Here's how the part is built. I have some questions about the finished solid (model axes, mm). Face numbers are marked on the shaded views. A direction names the side the tool comes from. Coordinates: 2 decimals unless noted, no trailing zeros. Write each loop counter-clockwise with the first axis right and the second up, starting at its lowest first coordinate (ties: lowest second). Pieces come first, ordered by that corner, then holes. Notation, with made-up numbers: (28, 52) -> (60, 52) arc R26 cw to (60, 68) -> close; hole circle Ø6 at (-25, -1.75). An arc over 180 degrees is marked (long way). Use a Markdown table: item, result. Add a question column.
Item 1: Imagine slicing it at C-C, the plane z = 17. Write out the boundary of the cut face in (x, y), and give its area (3 significant figures).
Item 2: If I drill on line 1 along Y through (x, z) = (13.5, 2.05); line 2 along Z through (x, y) = (-10.5, 32); line 3 along X through (y, z) = (31.5, 4), over which ranges is the centre line in solid material (lowest first)? Write a range as from..to.
Item 3: Imagine slicing it at B-B, the plane x = 10. Write out the boundary of the cut face in (y, z), and give its area (3 significant figures).
Item 4: On a 3-axis mill with a long thin cutter (end or side, diameter ignored), from which of +Z, -Z, +X, -X, +Y, -Y can I reach the whole of each face in a straight line? I mean the marked faces 1 and 2. Say none if no direction works.
Item 5: Imagine slicing it at D-D, the plane z = 5. Write out the boundary of the cut face in (x, y).
Item 6: Imagine slicing it at A-A, the plane y = 42. Write out the boundary of the cut face in (x, z), and give its area (3 significant figures).
Item 7: Will these pins go through, and if not, where does the flat tip stop? pin 1 Ø1.4 at (x, y) = (7.5, 17) entering from -Z; pin 2 Ø4.5 at (x, y) = (-13.5, 0) entering from +Z; pin 3 Ø0.6 at (x, z) = (18.5, 11.5) entering from -Y; pin 4 Ø5 at (x, z) = (5, 8) entering from -Y.
```python
from build123d import *

# Parameters (mm, degrees)
SKETCH1_R           = 1.65
BOSS_EXTRUDE1_DEPTH = 3
BOSS_EXTRUDE2_DEPTH = 40
CHAMFER1_SIZE       = 3
CUT_EXTRUDE3_START  = -29
SKETCH4_W           = 14.985281374
SKETCH4_H           = 16.743157806
SKETCH4_W_2         = 6.029437252
CUT_EXTRUDE3_DEPTH  = 29
CUT_EXTRUDE4_DEPTH  = 86
CUT_EXTRUDE5_DEPTH  = 6


with BuildPart() as part:
    # Sketch1 → Boss-Extrude1 (new body)
    with BuildSketch(Plane.XY):
        Polygon((-20, 104), (-20, -4), (-9.014718626, -4), (-5.014718626, 0), (5.014718626, 0), (9.014718626, -4), (20, -4), (20, 104), (9.014718626, 104), (5.014718626, 100), (-5.014718626, 100), (-9.014718626, 104), align=None)
        with Locations((-13.5, 100)):
            Circle(SKETCH1_R, mode=Mode.SUBTRACT)
        with Locations((-13.5, 0)):
            Circle(SKETCH1_R, mode=Mode.SUBTRACT)
        with Locations(Location((13.5, 0, 0), (0, 0, 180))):
            Circle(SKETCH1_R, mode=Mode.SUBTRACT)
        with Locations(Location((13.5, 100, 0), (0, 0, 180))):
            Circle(SKETCH1_R, mode=Mode.SUBTRACT)
    extrude(amount=BOSS_EXTRUDE1_DEPTH)

    # Sketch2 → Boss-Extrude2 (add, through all)
    with BuildSketch(Plane.ZY.offset(20)):
        Polygon((3, 0), (32, 16.743157806), (32, 49.770526581), (3, 100), align=None)
    extrude(amount=-BOSS_EXTRUDE2_DEPTH)

    # Chamfer1
    chamfer1_edges = [part.edges().sort_by_distance(p)[0] for p in [
        (20, 33.256842194, 32),
        (-20, 33.256842194, 32),
    ]]
    chamfer(chamfer1_edges, length=CHAMFER1_SIZE)

    # Sketch4 → Cut-Extrude3 (cut)
    with BuildSketch(Plane.XY.offset(32).offset(CUT_EXTRUDE3_START)):
        with Locations((-12.507359313, 8.371578903)):
            Rectangle(SKETCH4_W, SKETCH4_H)
        with Locations((12.507359313, 8.371578903)):
            Rectangle(SKETCH4_W, SKETCH4_H)
        with Locations((0, 8.371578903)):
            Rectangle(SKETCH4_W_2, SKETCH4_H)
    extrude(amount=CUT_EXTRUDE3_DEPTH, mode=Mode.SUBTRACT)

    # Sketch5 → Cut-Extrude4 (cut)
    with BuildSketch(Plane(origin=(0, 104, 0), x_dir=(1, 0, 0), z_dir=(0, 1, 0))):
        Polygon((18, -3), (18, -28.171572875), (16.171572875, -30), (-16.171572875, -30), (-18, -28.171572875), (-18, -3), align=None)
    extrude(amount=-CUT_EXTRUDE4_DEPTH, mode=Mode.SUBTRACT)

    # Sketch6 → Cut-Extrude5 (cut)
    with BuildSketch(Plane(origin=(0, 16.743157806, 0), x_dir=(-1, 0, 0), z_dir=(0, -1, 0))):
        Polygon((5.014718626, -29), (15.757359313, -29), (18.757359313, -26), (20.757359313, -26), (20.757359313, -3), (5.014718626, -3), align=None)
        Polygon((-5.014718626, -3), (-5.014718626, -29), (-15.757359313, -29), (-18.757359313, -26), (-20.757359313, -26), (-20.757359313, -3), align=None)
    extrude(amount=-CUT_EXTRUDE5_DEPTH, mode=Mode.SUBTRACT)


solid = part.part
```
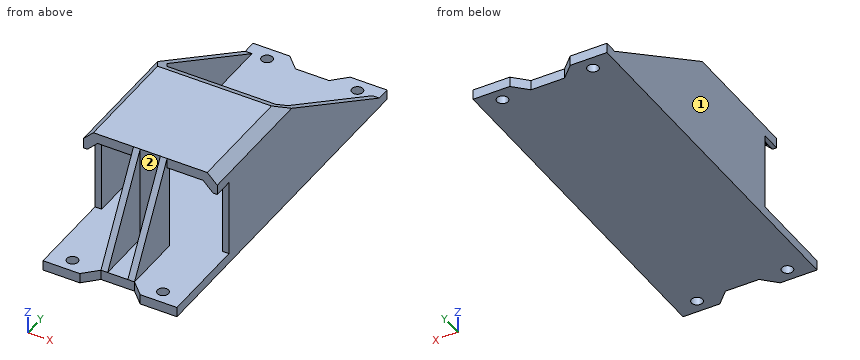
Ans:
| question | item | result |
|---|---|---|
| 1 | outline | (-20, 22.74) -> (-18, 22.74) -> (-18, 75.75) -> (-20, 75.75) -> close; (-5.01, 8.08) -> (-3.01, 8.08) -> (-3.01, 16.74) -> (3.01, 16.74) -> (3.01, 8.08) -> (5.01, 8.08) -> (5.01, 18) -> (-5.01, 18) -> close; (18, 22.74) -> (20, 22.74) -> (20, 75.75) -> (18, 75.75) -> close |
| 1 | area | 259 mm^2 |
| 2 | line 1 | y = -4..-1.65, 1.65..98.35, 101.65..104 |
| 2 | line 2 | z = 0..3, 30..32 |
| 2 | line 3 | x = -20..-18, 18..20 |
| 3 | outline | (-4, 0) -> (104, 0) -> (104, 3) -> (-4, 3) -> close; (16.74, 29) -> (18, 29) -> (18, 30) -> (53.23, 30) -> (49.77, 32) -> (16.74, 32) -> close |
| 3 | area | 395 mm^2 |
| 4 | face 1 | +Z, -Z, -X, +Y, -Y |
| 4 | face 2 | +Z, -Y |
| 5 | outline | (-20, 22.74) -> (-18, 22.74) -> (-18, 96.54) -> (-20, 96.54) -> close; (-5.01, 1.15) -> (-3.01, 1.15) -> (-3.01, 16.74) -> (3.01, 16.74) -> (3.01, 1.15) -> (5.01, 1.15) -> (5.01, 18) -> (-5.01, 18) -> close; (18, 22.74) -> (20, 22.74) -> (20, 96.54) -> (18, 96.54) -> close |
| 6 | outline | (-20, 0) -> (20, 0) -> (20, 29) -> (17, 32) -> (-17, 32) -> (-20, 29) -> close; hole (-18, 3) -> (18, 3) -> (18, 28.17) -> (16.17, 30) -> (-16.17, 30) -> (-18, 28.17) -> close |
| 6 | area | 302 mm^2 |
| 7 | pin 1 | stops at z = 0 |
| 7 | pin 2 | stops at z = 3 |
| 7 | pin 3 | stops at y = 22.74 |
| 7 | pin 4 | stops at y = 1.44 |
